```python
from build123d import *

# Parameters (mm, degrees)
EXTRUDE_1_DEPTH      = 1
EXTRUDE_1_DEPTH_BACK = 1
CHAMFER_2_SIZE       = 5


with BuildPart() as part:
    # Эскиз1 → Бобышка-Вытянуть1 (new, two sides: drawn at the far end of the back side and taken through both)
    with BuildSketch(Plane(origin=(0, 0, 0), x_dir=(1, 0, 0), z_dir=(0, 1, 0)).offset(-EXTRUDE_1_DEPTH_BACK)):
        Polygon((5, 52), (82, 22), (82, 0), (0, 0), (0, 52), align=None)
    extrude(amount=EXTRUDE_1_DEPTH + EXTRUDE_1_DEPTH_BACK)

    # Фаска2
    chamfer_2_edges = [part.edges().sort_by_distance(p)[0] for p in [
        (0, 0, 0),
        (82, 0, 0),
    ]]
    chamfer(chamfer_2_edges, length=CHAMFER_2_SIZE)


solid = part.part
```
Geometry check sheet. Reference: the model listing, model coordinates, mm. Coordinates: 2 decimals unless noted, no trailing zeros. Order: outer loops, then holes, each group sorted by start corner. A loop starts at its lowest first (then second) coordinate and runs counter-clockwise, first axis right, second up. Notation, with made-up numbers: (27, 11) - (43, 11) arc R20 ccw to (43, 15) - close; hole circle Ø8 at (-15.5, 8.5). An arc over 180 degrees is marked (long way). Answer in a Markdown table with one row per item. Add a question column.
1. Material ranges on L1, parallel to Z at x = 53, y = 0.7; L2, parallel to Z at x = 76, y = 0.8; L3, parallel to X at y = -0.3, z = -3.5, recorded low to high. Write a range as [from, to].
2. Section check C-C (x = 42). Enter the section's corners in (y, z).
3. Section check B-B (z = -31). Enter the section's corners in (x, y), plus the area to 3 significant figures.
4. Section check A-A (y = -0.1). Enter the section's corners in (x, z).
Data:
| question | item | result |
|---|---|---|
| 1 | L1 | z = [-33.3, 0] |
| 1 | L2 | z = [-24.34, 0] |
| 1 | L3 | x = [1.5, 80.5] |
| 2 | outline | (-1, -37.58) - (1, -37.58) - (1, 0) - (-1, 0) - close |
| 3 | outline | (0, -1) - (58.9, -1) - (58.9, 1) - (0, 1) - close |
| 3 | area | 118 mm² |
| 4 | outline | (0, -52) - (5, -52) - (82, -22) - (82, -5) - (77, 0) - (5, 0) - (0, -5) - close |
